from build123d import *

# Parameters (mm, degrees)
SKETCH_1_R          = 6.75
SKETCH_1_R_2        = 1.6
EXTRUDE_1_DEPTH     = 3
SKETCH_2_R          = 1.6
CUT_EXTRUDE_1_DEPTH = 10
SKETCH_3_W          = 59.008256567
SKETCH_3_H          = 13.932505023
CUT_EXTRUDE_2_DEPTH = 57.71860365
FILLET_1_R          = 2


with BuildPart() as part:
    # 草图1 → 凸台-拉伸1 (new body)
    with BuildSketch(Plane.XY):
        with BuildLine():
            Line((2, 0), (36, 0))
            ThreePointArc((36, 0), (37.414213562, -0.585786438), (38, -2))
            Line((38, -2), (38, -40))
            ThreePointArc((38, -40), (37.414213562, -41.414213562), (36, -42))
            Line((36, -42), (2, -42))
            ThreePointArc((2, -42), (0.585786438, -41.414213562), (0, -40))
            Line((0, -40), (0, -2))
            ThreePointArc((0, -2), (0.585786438, -0.585786438), (2, 0))
        make_face()
        with Locations((19, -21)):
            Circle(SKETCH_1_R, mode=Mode.SUBTRACT)
        with Locations((19, -11.5)):
            Circle(SKETCH_1_R_2, mode=Mode.SUBTRACT)
        with Locations((27.227241336, -25.75)):
            Circle(SKETCH_1_R_2, mode=Mode.SUBTRACT)
        with Locations((10.772758664, -25.75)):
            Circle(SKETCH_1_R_2, mode=Mode.SUBTRACT)
    extrude(amount=EXTRUDE_1_DEPTH)

    # 草图2 → 切除-拉伸1 (cut)
    with BuildSketch(Plane(origin=(0, 0, 0), x_dir=(-1, 0, 0), z_dir=(0, 0, -1))):
        with Locations((-13, -38)):
            Circle(SKETCH_2_R)
        with Locations((-25, -38)):
            Circle(SKETCH_2_R)
    extrude(amount=-CUT_EXTRUDE_1_DEPTH, mode=Mode.SUBTRACT)

    # 草图3 → 切除-拉伸2 (cut, through all)
    with BuildSketch(Plane.XY.offset(3)):
        with Locations((20.753628174, -0.033747488)):
            Rectangle(SKETCH_3_W, SKETCH_3_H)
    extrude(amount=-CUT_EXTRUDE_2_DEPTH, mode=Mode.SUBTRACT)

    # 圆角1
    fillet_1_edges = [part.edges().sort_by_distance(p)[0] for p in [
        (38, -7, 1.5),
        (0, -7, 1.5),
    ]]
    fillet(fillet_1_edges, radius=FILLET_1_R)


solid = part.part
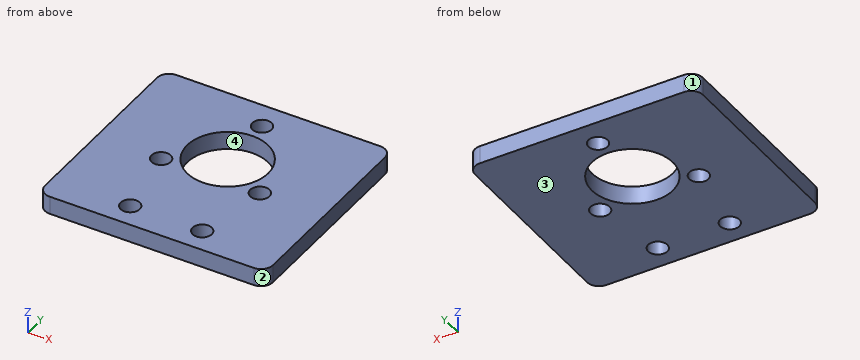
The model under review builds one solid part; all positions refer to its coordinate system, in mm. Face numbers are marked on the shaded views. Give positions to 0.01 mm unless a question says otherwise; leave off trailing zeros. Order: outer loops, then holes, each group sorted by start corner. A loop starts at its lowest first (then second) coordinate and runs counter-clockwise, first axis right, second up. Notation, with made-up numbers: (72.25, 59.25) -> (109.25, 59.25) arc R24 ccw to (109.25, 84.25) -> close; hole circle Ø11 at (-0.5, -4.75). An arc over 180 degrees is marked (long way). Write item = value, one per line. Start each with the question number.
(1) For L1, parallel to Y at x = 19, z = 1; L2, parallel to Y at x = 13.5, z = 1; L3, parallel to X at y = -27, z = 1.55, list the stretches that pass through material, from the lowest coordinate up. Write a range as from..to.
(2) Take a section at B-B (z = 1.8). Write out the cut boundary in (x, y).
(3) Take a section at A-A (x = 19). Write out the cut boundary in (y, z), plus the area to 3 significant figures.
(4) For pin 1 Ø2.5 at (x, y) = (10.77, -25.75) entering from +Z; pin 2 Ø3.5 at (x, y) = (19, -11.5) entering from -Z, all flat-tipped, find the tip position at first contact; note any pin that passes through.
(5) Draft analysis for pull direction X (two halves, no side actions). For the marked faces 1, 2, 3 and 4, state which applies: +X half, -X half, draft (parallel to the pull), parting line (faces both ways), or undercut.
(6) Take a section at C-C (y = -25.75). Write out the cut boundary in (x, z).
(7) Take a section at D-D (y = -18). Write out the cut boundary in (x, z), plus the area to 3 significant figures.
Returned:
q1.L1 = -42..-27.75, -14.25..-13.1, -9.9..-7
q1.L2 = -42..-39.52, -36.48..-24.91, -17.09..-7
q1.L3 = 0..9.77, 11.77..15.91, 22.09..26.23, 28.23..38
q2.outline = (0, -40) arc R2 ccw to (2, -42) -> (36, -42) arc R2 ccw to (38, -40) -> (38, -9) arc R2 ccw to (36, -7) -> (2, -7) arc R2 ccw to (0, -9) -> close; hole circle Ø3.2 at (10.77, -25.75); hole circle Ø3.2 at (13, -38); hole circle Ø13.5 at (19, -21); hole circle Ø3.2 at (19, -11.5); hole circle Ø3.2 at (25, -38); hole circle Ø3.2 at (27.23, -25.75)
q3.outline = (-42, 0) -> (-27.75, 0) -> (-27.75, 3) -> (-42, 3) -> close; (-14.25, 0) -> (-13.1, 0) -> (-13.1, 3) -> (-14.25, 3) -> close; (-9.9, 0) -> (-7, 0) -> (-7, 3) -> (-9.9, 3) -> close
q3.area = 54.9 mm²
q4.pin_1 = through
q4.pin_2 = 0
q5.face_1 = -X half
q5.face_2 = +X half
q5.face_3 = draft
q5.face_4 = undercut
q6.outline = (0, 0) -> (9.17, 0) -> (9.17, 3) -> (0, 3) -> close; (12.37, 0) -> (14.2, 0) -> (14.2, 3) -> (12.37, 3) -> close; (23.8, 0) -> (25.63, 0) -> (25.63, 3) -> (23.8, 3) -> close; (28.83, 0) -> (38, 0) -> (38, 3) -> (28.83, 3) -> close
q7.outline = (0, 0) -> (12.95, 0) -> (12.95, 3) -> (0, 3) -> close; (25.05, 0) -> (38, 0) -> (38, 3) -> (25.05, 3) -> close
q7.area = 77.7 mm²
